from build123d import *

# Parameters (mm, degrees)
SKETCH_1_W          = 150
SKETCH_1_H          = 110
EXTRUDE_1_DEPTH     = 15
SKETCH_2_R          = 38.5
EXTRUDE_2_DEPTH     = 100
SKETCH_4_R          = 29
CUT_EXTRUDE_1_DEPTH = 145
SKETCH_5_R          = 33
EXTRUDE_3_DEPTH     = 2
SKETCH_6_R          = 1.5
CUT_EXTRUDE_2_DEPTH = 2
SKETCH_7_R          = 38.5
SKETCH_7_R_2        = 33
EXTRUDE_4_DEPTH     = 22
SKETCH_8_R          = 10.643046967
CUT_EXTRUDE_3_DEPTH = 10


with BuildPart() as part:
    # 草图1 → 凸台-拉伸1 (new body)
    with BuildSketch(Plane.XY):
        Rectangle(SKETCH_1_W, SKETCH_1_H)
    extrude(amount=EXTRUDE_1_DEPTH)

    # 草图2 → 凸台-拉伸2 (add)
    with BuildSketch(Plane.XY.offset(15)):
        Circle(SKETCH_2_R)
    extrude(amount=EXTRUDE_2_DEPTH)

    # 草图4 → 切除-拉伸1 (cut)
    with BuildSketch(Plane.XY.offset(115)):
        Circle(SKETCH_4_R)
    extrude(amount=-CUT_EXTRUDE_1_DEPTH, mode=Mode.SUBTRACT)

    # 草图5 → 凸台-拉伸3 (add)
    with BuildSketch(Plane.XY.offset(115)):
        Circle(SKETCH_5_R)
    extrude(amount=EXTRUDE_3_DEPTH)

    # 草图6 → 切除-拉伸2 (cut)
    with BuildSketch(Plane.XY.offset(117)):
        with Locations((17.5, 0)):
            Circle(SKETCH_6_R)
        with Locations((-8.75, -15.155444566)):
            Circle(SKETCH_6_R)
        with Locations((-8.75, 15.155444566)):
            Circle(SKETCH_6_R)
    extrude(amount=-CUT_EXTRUDE_2_DEPTH, mode=Mode.SUBTRACT)

    # 草图7 → 凸台-拉伸4 (add)
    with BuildSketch(Plane.XY.offset(115)):
        Circle(SKETCH_7_R)
        Circle(SKETCH_7_R_2, mode=Mode.SUBTRACT)
    extrude(amount=EXTRUDE_4_DEPTH)

    # 草图8 → 切除-拉伸3 (cut)
    with BuildSketch(Plane.XY.offset(117)):
        with Locations((-22.11085185, 0)):
            Circle(SKETCH_8_R)
    extrude(amount=-CUT_EXTRUDE_3_DEPTH, mode=Mode.SUBTRACT)


solid = part.part
Could you check a few things on this model? Use its own coordinates, in mm. A direction names the side the tool comes from. Give positions to 0.01 mm unless a question says otherwise; leave off trailing zeros. Order: outer loops, then holes, each group sorted by start corner. A loop starts at its lowest first (then second) coordinate and runs counter-clockwise, first axis right, second up. Notation, with made-up numbers: M 43.25,-10.5 L 71.25,-10.5 A21 cw 71.25,2.5 Z; hole C 32,18 d4. An arc over 180 degrees is marked long. One line per question, with ' | ' between items.
1. If I drill on line 1 (Y direction, x = 0, z = 80); line 2 (Z direction, x = -63, y = 26.5); line 3 (Y direction, x = -14, z = 130), over which ranges is the centre line in solid material (lowest first)?
Results:
line 1: -38.5 to -29, 29 to 38.5 | line 2: 0 to 15 | line 3: -35.86 to -29.88, 29.88 to 35.86
2. I want a section at A-A (x = 0). List the corners of the cut face in (y, z) for me.
Results:
outline: M -55,0 L -29,0 L -29,115 L 29,115 L 29,0 L 55,0 L 55,15 L 38.5,15 L 38.5,137 L 33,137 L 33,117 L -33,117 L -33,137 L -38.5,137 L -38.5,15 L -55,15 Z
3. I want a section at D-D (y = -43). List the corners of the cut face in (x, z) for me.
Results:
outline: M -75,0 L 75,0 L 75,15 L -75,15 Z
4. I want a section at B-B (y = -4). List the corners of the cut face in (x, z) for me, and give its area (3 significant figures).
Results:
outline: M -75,0 L -28.72,0 L -28.72,107 L -31.97,107 L -31.97,117 L -32.76,117 L -32.76,137 L -38.29,137 L -38.29,15 L -75,15 Z; M -12.25,115 L 28.72,115 L 28.72,0 L 75,0 L 75,15 L 38.29,15 L 38.29,137 L 32.76,137 L 32.76,117 L -12.25,117 Z | area: 3,610 mm²
5. I want a section at C-C (z = 9). List the corners of the cut face in (x, y) for me, and give its area (3 significant figures).
Results:
outline: M -75,-55 L 75,-55 L 75,55 L -75,55 Z; hole C 0,0 d58 | area: 13,900 mm²
6. I'm going to push flat-ended pins straight in: pin 1 (6 mm diameter, centred on x = 20, z = 27.5, fed in from +Y); pin 2 (5 mm diameter, centred on x = -33.5, z = 91, fed in from -Y); pin 3 (1.8 mm diameter, centred on x = 17.5, y = 0, fed in from +Z); pin 4 (10 mm diameter, centred on x = -42, y = 36.5, fed in from -Z). Where does each tip first touch, or does it pass through?
Results:
pin 1: y = 34.54 | pin 2: y = -22.83 | pin 3: through | pin 4: z = 0
7. We'd pull the mould along X, two halves only. Please class faces 1 (the face through (-18, 37, 15)), 2 (the face through (-75, -1, 7)), 3 (the face through (-30, 0, 107)), 4 (the face through (-32.744, 0.468, 113.181)): +X half, -X half, draft (parallel to the pull), parting line (faces both ways), or undercut.
Results:
face 1: draft | face 2: -X half | face 3: undercut | face 4: undercut
8. For faces 5 (the face through (-1, 55, 7)), 6 (the face through (0, 0, 115)), 7 (the face through (7, 0, 117)), which set-ups out of +Z, -Z, +X, -X, +Y, -Y let a thin tool reach every point of the face, with its end or its side?
Results:
face 5: +Z, -Z, +X, -X, +Y | face 6: -Z | face 7: +Z
